Could you check a few things on this model? Use its own coordinates, in mm. Give positions to 0.01 mm unless a question says otherwise; leave off trailing zeros. Loops run counter-clockwise (first coordinate to the right, second up) from the corner with the lowest first, then second, coordinate; pieces in that order, holes last. Notation, with made-up numbers: M 22,10 L 37,10 A27 cw 37,34 Z; hole C 35.25,14 d11. An arc over 180 degrees is marked long. Answer in a Markdown table with one row per item. Add a question column.
1. I'm going to push flat-ended pins straight in: pin 1 Ø1 at (x, y) = (133.5, -4) entering from -Z; pin 2 Ø5 at (x, y) = (39, 4) entering from -Z. Where does each tip first touch, or does it pass through?
2. If we section it at A-A on x = 56.5: List the corners of the cut face in (y, z) for me.
3. If we section it at C-C on y = -1.25: List the corners of the cut face in (x, z) for me, then the cut area to 3 significant figures.
4. If we section it at B-B on z = 6: List the corners of the cut face in (x, y) for me.
5. I need wall thicknesses on line 1 along Z through (x, y) = (74.5, -3); line 2 along Z through (x, y) = (137, -5.25); line 3 along Y through (x, z) = (83.5, 4.25). Which ranges of each line are inside material? Lowest first, please. Write a range as from..to.
Autodesk Inventor part; units mm, degrees
ref_plane "YZ Plane" through (0, 0, 0) normal (1, 0, 0) x (0, 1, 0)
ref_plane "XZ Plane" through (0, 0, 0) normal (0, 1, 0) x (-1, 0, 0)
ref_plane "XY Plane" through (0, 0, 0) normal (0, 0, 1) x (1, 0, 0)
sketch "Sketch1" plane through (0, 0, 0) normal (1, 0, 0) x (0, 1, 0)
  circle A0 centre (0, 0) radius 6.35 construction
  line L0 (0, 0) -> (6.35, -3.6662) construction
  line L1 (0, 0) -> (7.3323, 0) construction
  line L2 (0, 0) -> (6.35, 3.6662) construction
  line L3 (0, 0) -> (7.3323, 0) construction
  line L4 (0, 0) -> (6.35, 3.6662) construction
  line L5 (0, 0) -> (0, 7.3323) construction
  line L6 (0, 0) -> (-6.35, 3.6662) construction
  line L7 (0, 0) -> (-6.35, -3.6662) construction
  line L8 (0, 0) -> (0, -7.3323) construction
  line L9 (0, 7.3323) -> (6.35, 3.6662)
  line L10 (6.35, 3.6662) -> (6.35, -3.6662)
  line L11 (6.35, -3.6662) -> (0, -7.3323)
  line L12 (0, -7.3323) -> (-6.35, -3.6662)
  line L13 (-6.35, -3.6662) -> (-6.35, 3.6662)
  line L14 (-6.35, 3.6662) -> (0, 7.3323)
  dimension "d0" = 12.7
  dimension "d1" = 30
  dimension "d2" = 30
  dimension "d5" = 360
extrude "Extrusion1" add sketch "Sketch1" along normal blind 152.4
properties part number "axle"
Results:
| question | item | result |
|---|---|---|
| 1 | pin 1 | z = -5.31 |
| 1 | pin 2 | z = -6.47 |
| 2 | outline | M -6.35,-3.67 L 0,-7.33 L 6.35,-3.67 L 6.35,3.67 L 0,7.33 L -6.35,3.67 Z |
| 3 | outline | M 0,-6.61 L 152.4,-6.61 L 152.4,6.61 L 0,6.61 Z |
| 3 | area | 2,010 mm2 |
| 4 | outline | M 0,-2.31 L 152.4,-2.31 L 152.4,2.31 L 0,2.31 Z |
| 5 | line 1 | -5.6..5.6 |
| 5 | line 2 | -4.3..4.3 |
| 5 | line 3 | -5.34..5.34 |
